Source: CAD feature listing. Evaluate the final solid. Frame: model axes, mm. A direction names the side the tool comes from. Coordinates: 2 decimals unless noted, no trailing zeros. Order: outer loops, then holes, each group sorted by start corner. A loop starts at its lowest first (then second) coordinate and runs counter-clockwise, first axis right, second up.
```python
from build123d import *

# Parameters (mm, degrees)
F0_W     = 35.2
F0_H     = 35.2
F1_DEPTH = 28
F2_R     = 11
F3_DEPTH = 2
F4_R     = 2.5
F5_DEPTH = 21
F7_D     = 2.5


with BuildPart() as f1:
    # F0 (on Top) → F1 (new body)
    with BuildSketch(Plane.XY):
        Rectangle(F0_W, F0_H)
    extrude(amount=F1_DEPTH)

    # F2 (on face) → F3 (join)
    with BuildSketch(Plane.XY.offset(28)):
        Circle(F2_R)
    extrude(amount=F3_DEPTH)

    # F4 (on face) → F5 (join)
    with BuildSketch(Plane.XY.offset(30)):
        Circle(F4_R)
    extrude(amount=F5_DEPTH)

    # F7 (through all)
    with Locations(Plane.XY.offset(28)):
        with Locations((13, 13), (13, -13), (-13, -13), (-13, 13)):
            Hole(F7_D / 2)


solid = f1.part
```
Q1. Set-up query: faces 4 (the cylindrical face through (-0.54, -2.44, 40.35)), 5 (the flat face through (0, -17.6, 14)). Return all of +Z, -Z, +X, -X, +Y, -Y with unobstructed straight access to the full face (end or side cutting, diameter ignored); none if empty.
Solutions:
face 4: +Z
face 5: +Z, -Z, +X, -X, -Y
Q2. Pin query (flat end, axial travel): P1, Ø1.5, axis at x = 3, z = 31.5, coming from the +Y side; P2, Ø1.5, axis at x = -3, y = -13.5, coming from the +Z side; P3, Ø6, axis at x = 11.5, y = -5, coming from the +Z side; P4, Ø2, axis at x = 13, y = 13, coming from the -Z side. Return the tip coordinate at first contact, or that it passes through.
Solutions:
P1: stops at y = 1.09
P2: stops at z = 28
P3: stops at z = 30
P4: passes through
Q3. Section query C-C on z = 11. Output: boundary loops of the cut face in (x, y).
Solutions:
outline: (-17.6, -17.6) - (17.6, -17.6) - (17.6, 17.6) - (-17.6, 17.6) - close; hole circle Ø2.5 at (-13, -13); hole circle Ø2.5 at (-13, 13); hole circle Ø2.5 at (13, -13); hole circle Ø2.5 at (13, 13)
Q4. Pull-direction query (X, two-part tool) for faces 1 (the flat face through (-8, 8, 28)), 2 (the flat face through (17.6, 0, 14)), 3 (the cylindrical face through (-12.84, -11.76, 13.8)); classes: pulls with the +X half, pulls with the -X half, needs draft (parallel to the pull), parting line crosses it, or undercut.
Solutions:
face 1: needs draft
face 2: pulls with the +X half
face 3: undercut
Q5. Section query D-D on x = 0. Output: boundary loops of the cut face in (y, z).
Solutions:
outline: (-17.6, 0) - (17.6, 0) - (17.6, 28) - (11, 28) - (11, 30) - (2.5, 30) - (2.5, 51) - (-2.5, 51) - (-2.5, 30) - (-11, 30) - (-11, 28) - (-17.6, 28) - close
Q6. Material intervals for line 1 along Y through (x, z) = (-13, 16.5); line 2 along Y through (x, z) = (14, 3.5), sorted ascending.
Solutions:
line 1: y = -17.6 to -14.25, -11.75 to 11.75, 14.25 to 17.6
line 2: y = -17.6 to -13.75, -12.25 to 12.25, 13.75 to 17.6
Q7. Section query A-A on x = -13. Output: boundary loops of the cut face in (y, z).
Solutions:
outline: (-17.6, 0) - (-14.25, 0) - (-14.25, 28) - (-17.6, 28) - close; (-11.75, 0) - (11.75, 0) - (11.75, 28) - (-11.75, 28) - close; (14.25, 0) - (17.6, 0) - (17.6, 28) - (14.25, 28) - close
